from build123d import *

# Parameters (mm, degrees)
F1_DEPTH = 10


with BuildPart() as f1:
    # F0 (on Front) → F1 (new body)
    with BuildSketch(Plane.XZ):
        Polygon((0, 35), (0, 0), (61.478138, 0), (80, 18.521862), (63.894674, 34.252785), (50, 20), (34.47455, 35), align=None)
    extrude(amount=F1_DEPTH)


solid = f1.part
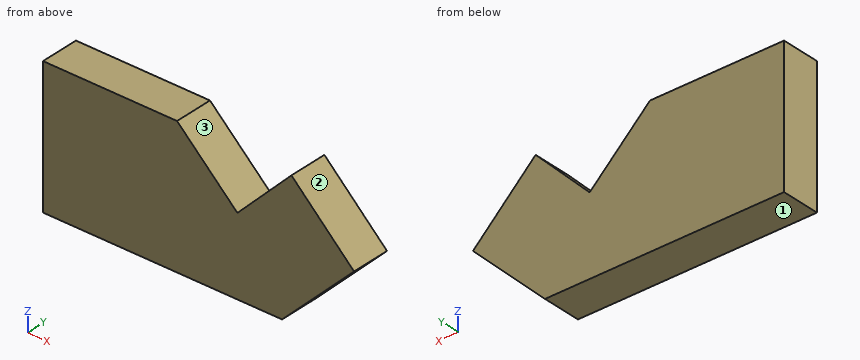
CAD build for the part. Positions are in the model's coordinates, mm. Face numbers are marked on the shaded views. Coordinates: 2 decimals unless noted, no trailing zeros. Write each loop counter-clockwise with the first axis right and the second up, starting at its lowest first coordinate (ties: lowest second). Pieces come first, ordered by that corner, then holes. Notation, with made-up numbers: (3, -35) - (55, -35) arc R28 ccw to (55, -7) - close; hole circle Ø1 at (45, 72.5). An arc over 180 degrees is marked (long way). Use a Markdown table: item, result. Add a question column.
Item 1: Band-saw the part on A-A, the plane y = -8.75. Give the cut face in (x, z).
Item 2: Mould opens along X. For the marked faces 1, 2 and 3 say: pulls with the +X half, pulls with the -X half, needs draft (parallel to the pull), parting line crosses it, or undercut.
Item 3: Band-saw the part on D-D, the plane x = 74.5. Give the cut face in (y, z), and give its area (3 significant figures).
Item 4: Drill centre lines: L1, parallel to Z at x = 50, y = -3; L2, parallel to X at y = -2.75, z = 32.5; L3, parallel to X at y = -5.5, z = 22. Where is each one in solid material? Low to high. Write a range as from..to.
Item 5: Band-saw the part on B-B, the plane z = 29. Give the cut face in (x, y), and give its area (3 significant figures).
Item 6: Band-saw the part on C-C, the plane z = 23.5. Give the cut face in (x, y).
Numbers:
| question | item | result |
|---|---|---|
| 1 | outline | (0, 0) - (61.48, 0) - (80, 18.52) - (63.89, 34.25) - (50, 20) - (34.47, 35) - (0, 35) - close |
| 2 | face 1 | needs draft |
| 2 | face 2 | pulls with the +X half |
| 2 | face 3 | undercut |
| 3 | outline | (-10, 13.02) - (0, 13.02) - (0, 23.89) - (-10, 23.89) - close |
| 3 | area | 109 mm2 |
| 4 | L1 | 0..20 |
| 4 | L2 | 0..37.06, 62.19..65.69 |
| 4 | L3 | 0..47.93, 51.95..76.44 |
| 5 | outline | (0, -10) - (40.68, -10) - (40.68, 0) - (0, 0) - close; (58.77, -10) - (69.27, -10) - (69.27, 0) - (58.77, 0) - close |
| 5 | area | 512 mm2 |
| 6 | outline | (0, -10) - (46.38, -10) - (46.38, 0) - (0, 0) - close; (53.41, -10) - (74.9, -10) - (74.9, 0) - (53.41, 0) - close |
